CAD build for the part. Positions are in the model's coordinates, mm. Face numbers are marked on the shaded views. Give positions to 0.01 mm unless a question says otherwise; leave off trailing zeros. Loops run counter-clockwise (first coordinate to the right, second up) from the corner with the lowest first, then second, coordinate; pieces in that order, holes last. Notation, with made-up numbers: (-17.5, 13.5) -> (23.5, 13.5) arc R34 ccw to (23.5, 51.5) -> close; hole circle Ø10 at (78, 65). An arc over 180 degrees is marked (long way). Use one line per item in the form item = value.
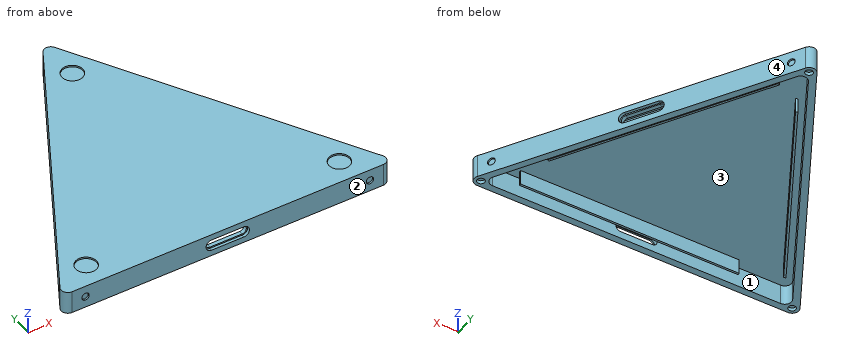
```python
from build123d import *

# Parameters (mm, degrees)
BOSS_EXTRU_1_DEPTH      = 15
BOSS_EXTRU_2_DEPTH      = 2
ESQUISSE3_W             = 163.463234946
ESQUISSE3_H             = 1.5
BOSS_EXTRU_3_DEPTH      = 11
ENL_V_MAT_EXTRU_1_DEPTH = 2.1
ENL_V_MAT_EXTRU_2_REACH = 253.952
CONG_1_R                = 5
ESQUISSE6_R             = 7.75
ENL_V_MAT_EXTRU_3_DEPTH = 1.24
ESQUISSE7_R             = 2.75
ENL_V_MAT_EXTRU_4_DEPTH = 1.24
ESQUISSE8_R             = 2.75
ENL_V_MAT_EXTRU_5_DEPTH = 2.48


with BuildPart() as part:
    # Esquisse1 → Boss.-Extru.1 (new body)
    with BuildSketch(Plane.XY):
        Polygon((-188.46822613, -62.203229112), (-63.46822613, 154.303121834), (61.53177387, -62.203229112), align=None)
        Polygon((52.871519833, -57.203229112), (-179.807972092, -57.203229112), (-63.46822613, 144.303121834), align=None, mode=Mode.SUBTRACT)
    extrude(amount=BOSS_EXTRU_1_DEPTH)

    # Esquisse2 → Boss.-Extru.2 (add)
    with BuildSketch(Plane.XY.offset(15)):
        Polygon((-63.46822613, 154.303121834), (-188.46822613, -62.203229112), (61.53177387, -62.203229112), align=None)
    extrude(amount=BOSS_EXTRU_2_DEPTH)

    # Esquisse3 → Boss.-Extru.3 (add)
    with BuildSketch(Plane(origin=(0, 0, 15), x_dir=(-1, 0, 0), z_dir=(0, 0, -1))):
        Polygon((55.550904435, 120.589918399), (-26.180713039, -20.97339565), (-24.881674933, -21.72339565), (56.84994254, 119.839918399), align=None)
        Polygon((162.980529474, -38.057243537), (161.681491369, -38.807243537), (79.949873895, 102.756070511), (81.248912001, 103.506070511), align=None)
        with Locations((54.104595722, -51.020446973)):
            Rectangle(ESQUISSE3_W, ESQUISSE3_H)
    extrude(amount=BOSS_EXTRU_3_DEPTH)

    # Esquisse4 → Enlèv. mat.-Extru.1 (cut)
    with BuildSketch(Plane(origin=(19.214042099, 11.093232378, 0), x_dir=(0, 0, -1), z_dir=(0.8660254037844387, 0.5000000000000001, 0))):
        with BuildLine():
            Line((-12.65, 52.464536457), (-12.65, 28.264536457))
            ThreePointArc((-12.65, 28.264536457), (-8.5, 24.114536457), (-4.35, 28.264536457))
            Line((-4.35, 28.264536457), (-4.35, 52.464536457))
            ThreePointArc((-4.35, 52.464536457), (-8.5, 56.614536457), (-12.65, 52.464536457))
        make_face()
    enl_v_mat_extru_1 = extrude(amount=-ENL_V_MAT_EXTRU_1_DEPTH, mode=Mode.SUBTRACT)

    # Esquisse5 → Enlèv. mat.-Extru.2 (cut, up to next)
    with BuildSketch(Plane(origin=(17.395388751, 10.043232378, 0), x_dir=(0, 0, -1), z_dir=(0.8660254037844386, 0.5000000000000003, 0)), mode=Mode.PRIVATE) as enl_v_mat_extru_2_sk1:
        with BuildLine():
            Line((-11.65, 52.464536457), (-11.65, 28.264536457))
            ThreePointArc((-11.65, 28.264536457), (-8.5, 25.114536457), (-5.35, 28.264536457))
            Line((-5.35, 28.264536457), (-5.35, 52.464536457))
            ThreePointArc((-5.35, 52.464536457), (-8.5, 55.614536457), (-11.65, 52.464536457))
        make_face()
    enl_v_mat_extru_2_tool1 = extrude(enl_v_mat_extru_2_sk1.sketch, amount=-ENL_V_MAT_EXTRU_2_REACH, mode=Mode.PRIVATE) & part.part
    enl_v_mat_extru_2 = enl_v_mat_extru_2_tool1.solids().sort_by_distance((-2.786879, 44.999946, 8.5))[0]
    add(enl_v_mat_extru_2, mode=Mode.SUBTRACT)

    # Congé1
    cong_1_edges = [part.edges().sort_by_distance(p)[0] for p in [
        (52.871519833, -57.203229112, 7.5),
        (-63.46822613, 144.303121834, 7.5),
        (-179.807972092, -57.203229112, 7.5),
        (-188.46822613, -62.203229112, 8.5),
        (-63.46822613, 154.303121834, 8.5),
        (61.53177387, -62.203229112, 8.5),
    ]]
    fillet(cong_1_edges, radius=CONG_1_R)

    # Symétrie1: Enlèv. mat.-Extru.1, Enlèv. mat.-Extru.2 across plane
    add(enl_v_mat_extru_1.mirror(Plane(origin=(-11.551844836, -20.008382178, 0), x_dir=(0, 0, 1), z_dir=(0.5000000000000001, 0.8660254037844386, 0))), mode=Mode.SUBTRACT)
    add(enl_v_mat_extru_2.mirror(Plane(origin=(-11.551844836, -20.008382178, 0), x_dir=(0, 0, 1), z_dir=(0.5000000000000001, 0.8660254037844386, 0))), mode=Mode.SUBTRACT)

    # Esquisse6 → Enlèv. mat.-Extru.3 (cut)
    with BuildSketch(Plane.XY.offset(17)):
        with Locations((-63.46822613, 119.303121834)):
            Circle(ESQUISSE6_R)
        with Locations(Location((-158.157336997, -44.703229112, 0), (0, 0, 180))):
            Circle(ESQUISSE6_R)
        with Locations((31.220884738, -44.703229112)):
            Circle(ESQUISSE6_R)
    extrude(amount=-ENL_V_MAT_EXTRU_3_DEPTH, mode=Mode.SUBTRACT)

    # Esquisse7 → Enlèv. mat.-Extru.4 (cut)
    with BuildSketch(Plane.XZ.offset(62.203229112)):
        with Locations((42.871519833, 8.5)):
            Circle(ESQUISSE7_R)
        with Locations(Location((-169.807972092, 8.5, 0), (0, 0, 180))):
            Circle(ESQUISSE7_R)
    enl_v_mat_extru_4 = extrude(amount=-ENL_V_MAT_EXTRU_4_DEPTH, mode=Mode.SUBTRACT)

    # Symétrie2: Enlèv. mat.-Extru.4 across plane
    add(enl_v_mat_extru_4.mirror(Plane(origin=(-11.551844836, -20.008382178, 0), x_dir=(0, 0, 1), z_dir=(0.5000000000000001, 0.8660254037844386, 0))), mode=Mode.SUBTRACT)

    # Symétrie3: Enlèv. mat.-Extru.4 across plane
    add(enl_v_mat_extru_4.mirror(Plane(origin=(-20.182268228, 34.956713983, 0), x_dir=(0, 0, 1), z_dir=(0.5000000000000001, -0.8660254037844387, 0))), mode=Mode.SUBTRACT)

    # Esquisse8 → Enlèv. mat.-Extru.5 (cut)
    with BuildSketch(Plane(origin=(0, 0, 0), x_dir=(-1, 0, 0), z_dir=(0, 0, -1))):
        with Locations((-52.871519833, -57.203229112)):
            Circle(ESQUISSE8_R)
        with Locations(Location((63.46822613, 144.303121834, 0), (0, 0, 180))):
            Circle(ESQUISSE8_R)
        with Locations((179.807972092, -57.203229112)):
            Circle(ESQUISSE8_R)
    extrude(amount=-ENL_V_MAT_EXTRU_5_DEPTH, mode=Mode.SUBTRACT)


solid = part.part
```
1. Cut at D-D, the plane y = 132.5. Write the cut outline in (x, z).
Result sheet:
outline = (-76.06, 0) -> (-70.28, 0) -> (-70.28, 15) -> (-56.65, 15) -> (-56.65, 0) -> (-50.88, 0) -> (-50.88, 17) -> (-76.06, 17) -> close
2. Cut at A-A, the plane y = -32. Write the cut outline in (x, z), then the cut area to 3 significant figures.
Result sheet:
outline = (-171.03, 0) -> (-165.26, 0) -> (-165.26, 15) -> (-159.48, 15) -> (-159.48, 4) -> (-157.75, 4) -> (-157.75, 15) -> (38.32, 15) -> (38.32, 0) -> (44.09, 0) -> (44.09, 17) -> (-171.03, 17) -> close
area = 623 mm^2
3. Drop flat-ended pins along their axis: P1, Ø1.6, axis at y = -51.5, z = 7.5, coming from the +X side; P2, Ø0.8, axis at y = -51, z = 11, coming from the -X side; P3, Ø8, axis at x = -145, z = 3, coming from the +Y side; P4, Ø16, axis at x = -5.5, y = 41, coming from the -Z side. Give the stop position or say it passes through.
Result sheet:
P1 = 55.81
P2 = -182.23
P3 = 20.01
P4 = 0
4. Cut at C-C, the plane z = 8.5. State how many separate pieces and enclosed holes the cut face has, then the cut area to 3 significant figures.
Result sheet:
separate_pieces = 5
enclosed_holes = 0
area = 4,000 mm^2
5. Mould opens along X. For the marked faces 1, 2, 3 and 4 say: pulls with the +X half, pulls with the -X half, needs draft (parallel to the pull), parting line crosses it, or undercut.
Result sheet:
face_1 = undercut
face_2 = needs draft
face_3 = undercut
face_4 = pulls with the +X half
6. Cut at B-B, the plane x = -99.5. Write the cut outline in (y, z), then the cut area to 3 significant figures.
Result sheet:
outline = (-62.2, 0) -> (-57.2, 0) -> (-57.2, 15) -> (-51.77, 15) -> (-51.77, 4) -> (-50.27, 4) -> (-50.27, 15) -> (68.89, 15) -> (68.89, 4) -> (71.89, 4) -> (71.89, 15) -> (81.89, 15) -> (81.89, 0) -> (91.89, 0) -> (91.89, 17) -> (-62.2, 17) -> close
area = 583 mm^2
7. Drill centre lines: line 1 (X direction, y = 82, z = 14.5); line 2 (Y direction, x = -96, z = 10); line 3 (Y direction, x = -91.5, z = 6.25). Where is each one in solid material? Low to high.
Result sheet:
line_1 = -105.21 to -99.44, -93.67 to -91.93, -35 to -33.27, -27.5 to -21.72
line_2 = -62.2 to -57.2, -51.77 to -50.27, 74.96 to 77.96, 87.96 to 97.96
line_3 = -62.2 to -57.2, -51.77 to -50.27, 82.75 to 85.75, 95.75 to 105.75
